Geometry: final body of the model. Coordinates: model frame, mm. Face numbers are marked on the shaded views. A direction names the side the tool comes from. Give positions to 0.01 mm unless a question says otherwise; leave off trailing zeros. Loops run counter-clockwise (first coordinate to the right, second up) from the corner with the lowest first, then second, coordinate; pieces in that order, holes last.
1. Material intervals for line 1 along X through (y, z) = (480, 853); line 2 along Z through (x, y) = (-915.5, 28); line 3 along Y through (x, z) = (-491, 842.5), sorted ascending.
2. Section B-B, the plane x = -1210. Output: boundary loops of the cut face in (y, z).
3. First-contact query: P1, Ø6, axis at x = -1019.5, y = 14.5, coming from the -Z side; P2, Ø5, axis at x = -667, y = 125, coming from the +Z side; P3, Ø3, axis at x = -305.5, z = 926.5, coming from the -Y side. Flat tips, straight axial feed; report the tip coordinate or a pass-through.
4. Access query for the marked faces 1, 2 and 3. Directions: +Z, -Z, +X, -X, +Y, -Y. A direction counts if a zero-diameter tool reaches every point of the face in a straight line with its end or side. Return the directions, or none.
5. Section A-A, the plane z = 283. Output: boundary loops of the cut face in (x, y), then the cut area to 3 significant figures.
6. Section C-C, the plane y = 560. Output: boundary loops of the cut face in (x, z).
7. Draft query along X for the marked faces 4, 5, 6 and 7. Return one class per face: +X half, -X half, draft (parallel to the pull), parting line (faces both ways), or undercut.
8. Section D-D, the plane y = 201.5. Output: boundary loops of the cut face in (x, z), then the cut area to 3 significant figures.
from build123d import *

# Parameters (mm, degrees)
SKETCH012_W      = 1860
SKETCH012_H      = 880
EXTRUDE019_DEPTH = 580
SKETCH011_W      = 1800
SKETCH011_H      = 850
EXTRUDE018_DEPTH = 20
SKETCH003_W      = 400
SKETCH003_H      = 300
EXTRUDE015_DEPTH = 20
SKETCH004_W      = 1900
SKETCH004_H      = 150
EXTRUDE017_DEPTH = 20
SKETCH_W         = 1900
SKETCH_H         = 900
EXTRUDE016_DEPTH = 600
EXTRUDE006_DEPTH = 400
EXTRUDE007_DEPTH = 440


with BuildPart() as extrude019:
    # Sketch012 → Extrude019 (new body)
    with BuildSketch(Plane.XZ):
        with Locations((930, 440)):
            Rectangle(SKETCH012_W, SKETCH012_H)
    extrude(amount=-EXTRUDE019_DEPTH)


with BuildPart() as extrude019_1:
    # Extrude019 placement: moved
    add(extrude019.part.moved(Location((20, 20, 0))))


with BuildPart() as obj1:
    # Sketch011 → Extrude018 (new body)
    with BuildSketch(Plane.XZ):
        with Locations((900, 425)):
            Rectangle(SKETCH011_W, SKETCH011_H)
    extrude(amount=-EXTRUDE018_DEPTH)


with BuildPart() as obj1_1:
    # Extrude018 placement: moved
    add(obj1.part.moved(Location((50, 0, 0))))


with BuildPart() as fusion016:
    # Sketch003 → Extrude015 (new body)
    with BuildSketch(Plane.XY):
        with Locations((200, 150)):
            Rectangle(SKETCH003_W, SKETCH003_H)
    extrude(amount=EXTRUDE015_DEPTH)


with BuildPart() as fusion016_1:
    # Extrude015 placement: moved
    add(fusion016.part.moved(Location((266.66, 80, 880))))

    # Fusion016: union Extrude019, obj1
    add(extrude019_1.part)
    add(obj1_1.part)


with BuildPart() as extrude017:
    # Sketch004 → Extrude017 (new body)
    with BuildSketch(Plane.XZ):
        with Locations((950, 75)):
            Rectangle(SKETCH004_W, SKETCH004_H)
    extrude(amount=EXTRUDE017_DEPTH)


with BuildPart() as extrude017_1:
    # Extrude017 placement: moved
    add(extrude017.part.moved(Location((0, 600, 900))))


with BuildPart() as cut013:
    # Sketch → Extrude016 (new body)
    with BuildSketch(Plane.XZ):
        with Locations((950, 450)):
            Rectangle(SKETCH_W, SKETCH_H)
    extrude(amount=-EXTRUDE016_DEPTH)

    # Fusion006: union Extrude017
    add(extrude017_1.part)

    # Cut013: cut Fusion016
    add(fusion016_1.part, mode=Mode.SUBTRACT)


with BuildPart() as extrude006:
    # Sketch006 → Extrude006 (new body)
    with BuildSketch(Plane.YZ):
        Polygon((0, 0), (300, 0), (300, -100), (200, -100), align=None)
    extrude(amount=EXTRUDE006_DEPTH)


with BuildPart() as obj2:
    # Sketch007 → Extrude007 (new body)
    with BuildSketch(Plane.YZ):
        Polygon((-40, 0), (320, 0), (320, -120), (200, -120), align=None)
    extrude(amount=EXTRUDE007_DEPTH)


with BuildPart() as obj2_1:
    # Extrude007 placement: moved
    add(obj2.part.moved(Location((-20, 0, 0))))

    # Cut006: cut Extrude006
    add(extrude006.part, mode=Mode.SUBTRACT)


with BuildPart() as obj2_2:
    # Cut006 placement: moved
    add(obj2_1.part.moved(Location((266.66, 80, 900))))

    # Fusion017: union Cut013
    add(cut013.part)


with BuildPart() as mirror001:
    # Mirror001: instance of obj2
    add(obj2_2.part.mirror(Plane(origin=(0, 0, 0), x_dir=(0, -1, 0), z_dir=(1, 0, 0))))


solid = mirror001.part
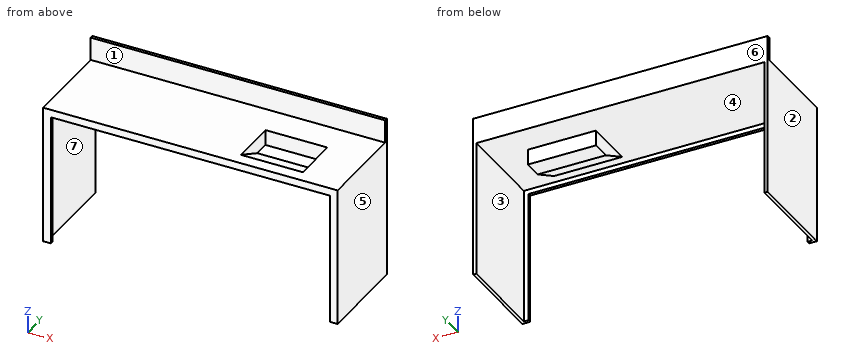
Answers below:
1. line 1: x = -1900 to -1880, -20 to 0
1. line 2: z = 880 to 900
1. line 3: y = 155 to 195, 380 to 400
2. outline: (0, 850) - (20, 850) - (20, 880) - (600, 880) - (600, 1050) - (580, 1050) - (580, 900) - (0, 900) - close
3. P1: stops at z = 850
3. P2: stops at z = 900
3. P3: stops at y = 580
4. face 1: +Z, +X, -X, -Y
4. face 2: +Z, -Z, -X, +Y, -Y
4. face 3: -Z, +Y
5. outline: (-1900, 0) - (-1850, 0) - (-1850, 20) - (-1880, 20) - (-1880, 600) - (-1900, 600) - close; (-50, 0) - (0, 0) - (0, 600) - (-20, 600) - (-20, 20) - (-50, 20) - close
5. area: 25,200 mm2
6. outline: (-1900, 0) - (-1880, 0) - (-1880, 880) - (-20, 880) - (-20, 0) - (0, 0) - (0, 900) - (-1900, 900) - close
7. face 4: undercut
7. face 5: +X half
7. face 6: draft
7. face 7: undercut
8. outline: (-1900, 0) - (-1880, 0) - (-1880, 880) - (-686.66, 880) - (-686.66, 819.25) - (-246.66, 819.25) - (-246.66, 880) - (-20, 880) - (-20, 0) - (0, 0) - (0, 900) - (-266.66, 900) - (-266.66, 839.25) - (-666.66, 839.25) - (-666.66, 900) - (-1900, 900) - close
8. area: 75,600 mm2
